from build123d import *

# Parameters (mm, degrees)
F1_DEPTH = 1.8
F2_R     = 0.5
F3_SIZE  = 0.5


with BuildPart() as f1:
    # F0 (on Top) → F1 (new body)
    with BuildSketch(Plane.XY):
        Polygon((-5.25, -15), (5.25, -15), (5.25, 15), (5.25, 23), (2.25, 23), (2.25, 15), (-2.25, 15), (-2.25, 23), (-5.25, 23), (-5.25, 15), align=None)
    extrude(amount=F1_DEPTH)

    # F2
    f2_edges = [f1.edges().sort_by_distance(p)[0] for p in [
        (-2.25, 23, 0.9),
        (2.25, 23, 0.9),
        (0, 15, 1.8),
        (0, 15, 0),
    ]]
    fillet(f2_edges, radius=F2_R)

    # F3
    f3_edges = [f1.edges().sort_by_distance(p)[0] for p in [
        (0, -15, 1.8),
        (5.25, -15, 0.9),
        (0, -15, 0),
        (-5.25, -15, 0.9),
    ]]
    chamfer(f3_edges, length=F3_SIZE)


solid = f1.part
CAD build for the part. Positions are in the model's coordinates, mm. A direction names the side the tool comes from. Give positions to 0.01 mm unless a question says otherwise; leave off trailing zeros. Write each loop counter-clockwise with the first axis right and the second up, starting at its lowest first coordinate (ties: lowest second). Pieces come first, ordered by that corner, then holes. Notation, with made-up numbers: (6.5, -5.5) - (16.5, -5.5) arc R21 cw to (16.5, 11.5) - close; hole circle Ø4 at (-29.75, -9). An arc over 180 degrees is marked (long way). Put each result on its own line as item: value.
(1) Wall check: L1, parallel to X at y = 20.5, z = 1.35; L2, parallel to Y at x = 1.25, z = 1.15; L3, parallel to Y at x = -3.5, z = 0.4. Give the ranges that are in metal, low to high.
Working result:
L1: -5.25 to -2.25, 2.25 to 5.25
L2: -15 to 15
L3: -14.9 to 23
(2) Drop a flat-ended pin along its axis: pin 1 Ø0.6 at (x, z) = (0, 1) entering from +Y. Give the stop position or say it passes through.
Working result:
pin 1: y = 15
(3) Tool access for faces 4 (the flat face through (5.25, 4, 1)), 5 (the flat face through (0, 15, 1)): list every direction of +Z, -Z, +X, -X, +Y, -Y with a clear straight run to the whole face (end or side of a thin tool).
Working result:
face 4: +Z, -Z, +X, +Y, -Y
face 5: +Z, -Z, +Y
(4) Pull direction X, two halves, no side cores. Call faces 1 (the flat face through (2.25, 19, 1)), 2 (the flat face through (0, 5, 1.8)), 3 (the flat face through (-5.25, 5, 1)): released by +X, released by -X, zero draft, split by the parting line, or undercut.
Working result:
face 1: undercut
face 2: zero draft
face 3: released by -X
(5) Saw through at B-B (x = 0.75). List the corners of the cut face in (y, z), then the cut area to 3 significant figures.
Working result:
outline: (-15, 0.5) - (-14.5, 0) - (14.5, 0) arc R0.5 ccw to (15, 0.5) - (15, 1.3) arc R0.5 ccw to (14.5, 1.8) - (-14.5, 1.8) - (-15, 1.3) - close
area: 53.6 mm^2
(6) Saw through at A-A (z = 1). List the corners of the cut face in (x, y), then the cut area to 3 significant figures.
Working result:
outline: (-5.25, -14.5) - (-4.75, -15) - (4.75, -15) - (5.25, -14.5) - (5.25, 23) - (2.75, 23) arc R0.5 ccw to (2.25, 22.5) - (2.25, 15) - (-2.25, 15) - (-2.25, 22.5) arc R0.5 ccw to (-2.75, 23) - (-5.25, 23) - close
area: 363 mm^2
